```python
from build123d import *

# Parameters (mm, degrees)
ESQUISSE1_R         = 2.5
ESQUISSE1_R_2       = 2.313714448
BOSS_EXTRU_9_DEPTH  = 10
ESQUISSE1_31_W      = 3
ESQUISSE1_31_H      = 24.915622322
BOSS_EXTRU_10_DEPTH = 2
ESQUISSE1_32_R      = 2.5
ESQUISSE1_32_R_2    = 2.313714448
BOSS_EXTRU_11_DEPTH = 15
CONG_1_R            = 1
CONG_2_R            = 0.5


with BuildPart() as part:
    # Esquisse1 → Boss.-Extru.9 (new body)
    # profile 1 of 3: a face of its own
    with BuildSketch(Plane.XY):
        Polygon((-18.775986612, 46.025144014), (-18.775986612, 42.525144014), (-14.123920218, 42.525144014), (115.224013388, 42.525144014), (115.224013388, 52.525144014), (-14.123920218, 52.525144014), (-18.775986612, 52.525144014), (-18.775986612, 51.00961058), (-18.775986612, 49.025144014), (-13.775986612, 49.025144014), (-13.775986612, 46.025144014), align=None)
        with Locations((48.224013388, 47.525144014)):
            Circle(ESQUISSE1_R, mode=Mode.SUBTRACT)
    # profile 2 of 3: a face of its own
    with BuildSketch(Plane.XY):
        with BuildLine():
            ThreePointArc((124.090146574, -39.974855986), (121.331451242, -71.462379164), (115.224013388, -102.474855986))
            Line((115.224013388, -102.474855986), (115.224013388, -112.474855986))
            ThreePointArc((115.224013388, -112.474855986), (133.372740942, -29.974855986), (115.224013388, 52.525144014))
            Line((115.224013388, 52.525144014), (115.224013388, 42.525144014))
            ThreePointArc((115.224013388, 42.525144014), (120.975797216, 13.946843769), (123.882639826, -15.059233664))
            Line((123.882639826, -15.059233664), (124.791681137, -15.059233664))
            Line((124.791681137, -15.059233664), (124.791681137, -39.974855986))
            Line((124.791681137, -39.974855986), (124.090146574, -39.974855986))
        make_face()
        with Locations((128.863881441, -27.559233664)):
            Circle(ESQUISSE1_R_2, mode=Mode.SUBTRACT)
    # profile 3 of 3: a face of its own
    with BuildSketch(Plane.XY):
        Polygon((-18.775986612, -105.974855986), (-13.775986612, -105.974855986), (-13.775986612, -108.974855986), (-18.775986612, -108.974855986), (-18.787756311, -112.474855986), (115.224013388, -112.474855986), (115.224013388, -102.474855986), (-18.787756311, -102.474855986), align=None)
        with Locations((48.224013388, -107.474855986)):
            Circle(ESQUISSE1_R, mode=Mode.SUBTRACT)
    extrude(amount=BOSS_EXTRU_9_DEPTH)

    # Esquisse1_31 → Boss.-Extru.10 (add)
    with BuildSketch(Plane.XY):
        with Locations((123.291681137, -27.517044825)):
            Rectangle(ESQUISSE1_31_W, ESQUISSE1_31_H)
    extrude(amount=BOSS_EXTRU_10_DEPTH)

    # Esquisse1_32 → Boss.-Extru.11 (add)
    with BuildSketch(Plane.XY):
        with Locations((48.224013388, 47.525144014)):
            Circle(ESQUISSE1_32_R)
        with Locations((128.863881441, -27.559233664)):
            Circle(ESQUISSE1_32_R_2)
        with Locations((48.224013388, -107.474855986)):
            Circle(ESQUISSE1_32_R)
    extrude(amount=BOSS_EXTRU_11_DEPTH)

    # Cong_1
    cong_1_edges = [part.edges().sort_by_distance(p)[0] for p in [
        (45.724013388, 47.525144014, 15),
        (126.550166993, -27.559233664, 15),
        (45.724013388, -107.474855986, 15),
    ]]
    fillet(cong_1_edges, radius=CONG_1_R)

    # Cong_2
    cong_2_edges = [part.edges().sort_by_distance(p)[0] for p in [
        (121.791681137, -27.517044825, 0),
        (121.791681137, -27.517044825, 2),
    ]]
    fillet(cong_2_edges, radius=CONG_2_R)


solid = part.part
```
Geometry: final body of the model. Coordinates: model frame, mm. A direction names the side the tool comes from. Coordinates: 2 decimals unless noted, no trailing zeros. Order: outer loops, then holes, each group sorted by start corner. A loop starts at its lowest first (then second) coordinate and runs counter-clockwise, first axis right, second up.
Item 1: Section query B-B (x = 2.5). Output: boundary loops of the cut face in (y, z).
Answer:
outline: (-112.47, 0) - (-102.47, 0) - (-102.47, 10) - (-112.47, 10) - close; (42.53, 0) - (52.53, 0) - (52.53, 10) - (42.53, 10) - close
Item 2: Access query for faces 1 (the face through (124.792, -27, 6)), 2 (the face through (-18.776, 51, 5)), 3 (the face through (49, -102.475, 5)), 4 (the face through (127.03, -28.97, 11.97)), 5 (the face through (125, -30, 0)). Directions: +Z, -Z, +X, -X, +Y, -Y. A direction counts if a zero-diameter tool reaches every point of the face in a straight line with its end or side. Return the directions, or none.
Answer:
face 1: +Z, -X
face 2: +Z, -Z, -X, +Y, -Y
face 3: +Z, -Z, -X
face 4: +Z
face 5: -Z, +X, -X, +Y, -Y
Item 3: Material intervals for line 1 along Y through (x, z) = (30, 6.75); line 2 along X through (y, z) = (-31, 4); line 3 along X through (y, z) = (-32, 6), sorted ascending.
Answer:
line 1: y = -112.47 to -102.47, 42.53 to 52.53
line 2: x = 124.79 to 133.37
line 3: x = 124.79 to 133.36
Item 4: Contact query for flat-ended pins moving along their axis: P1, Ø1, axis at x = 60.5, z = 11, coming from the +Y side; P2, Ø0.8, axis at x = 123.5, y = -31, coming from the +Z side; P3, Ø0.9, axis at y = 47.5, z = 4, coming from the -X side; P4, Ø8, axis at y = -20.5, z = 2.5, coming from the -X side. Output: stop coordinate, or through.
Answer:
P1: passes through
P2: stops at z = 2
P3: stops at x = -13.78
P4: stops at x = 121.79
Item 5: Draft query along Y for faces 6 (the face through (121.393, -71.024, 4.93)), 7 (the face through (-18.776, 44, 5)), 8 (the face through (49.38, -109.69, 11.97)), 9 (the face through (133.37, -31.17, 4.93)). Return one class per face: released by +Y, released by -Y, zero draft, split by the parting line, or undercut.
Answer:
face 6: undercut
face 7: zero draft
face 8: undercut
face 9: split by the parting line
Item 6: Section query A-A (z = 4.5). Output: boundary loops of the cut face in (x, y), then the cut area to 3 significant figures.
Answer:
outline: (-18.79, -112.47) - (115.22, -112.47) arc R196.59 ccw to (115.22, 52.53) - (-18.78, 52.53) - (-18.78, 49.03) - (-13.78, 49.03) - (-13.78, 46.03) - (-18.78, 46.03) - (-18.78, 42.53) - (115.22, 42.53) arc R295.39 cw to (123.88, -15.06) - (124.79, -15.06) - (124.79, -39.97) - (124.09, -39.97) arc R295.39 cw to (115.22, -102.47) - (-18.79, -102.47) - (-18.78, -105.97) - (-13.78, -105.97) - (-13.78, -108.97) - (-18.78, -108.97) - close
area: 3,770 mm2
Item 7: Section query D-D (y = -52). Output: boundary loops of the cut face in (x, z), then the cut area to 3 significant figures.
Answer:
outline: (123.44, 0) - (132.14, 0) - (132.14, 10) - (123.44, 10) - close
area: 87.0 mm2
Item 8: Section query C-C (y = -19). Output: boundary loops of the cut face in (x, z), then the cut area to 3 significant figures.
Answer:
outline: (121.79, 0.5) arc R0.5 ccw to (122.29, 0) - (133.07, 0) - (133.07, 10) - (124.79, 10) - (124.79, 2) - (122.29, 2) arc R0.5 ccw to (121.79, 1.5) - close
area: 88.6 mm2
